Could you check a few things on this drawing? It's one solid part, dimensions in mm from its lowest x, y, z. A direction names the side the tool comes from. Give positions to 0.01 mm unless a question says otherwise; leave off trailing zeros. Order: outer loops, then holes, each group sorted by start corner. A loop starts at its lowest first (then second) coordinate and runs counter-clockwise, first axis right, second up.
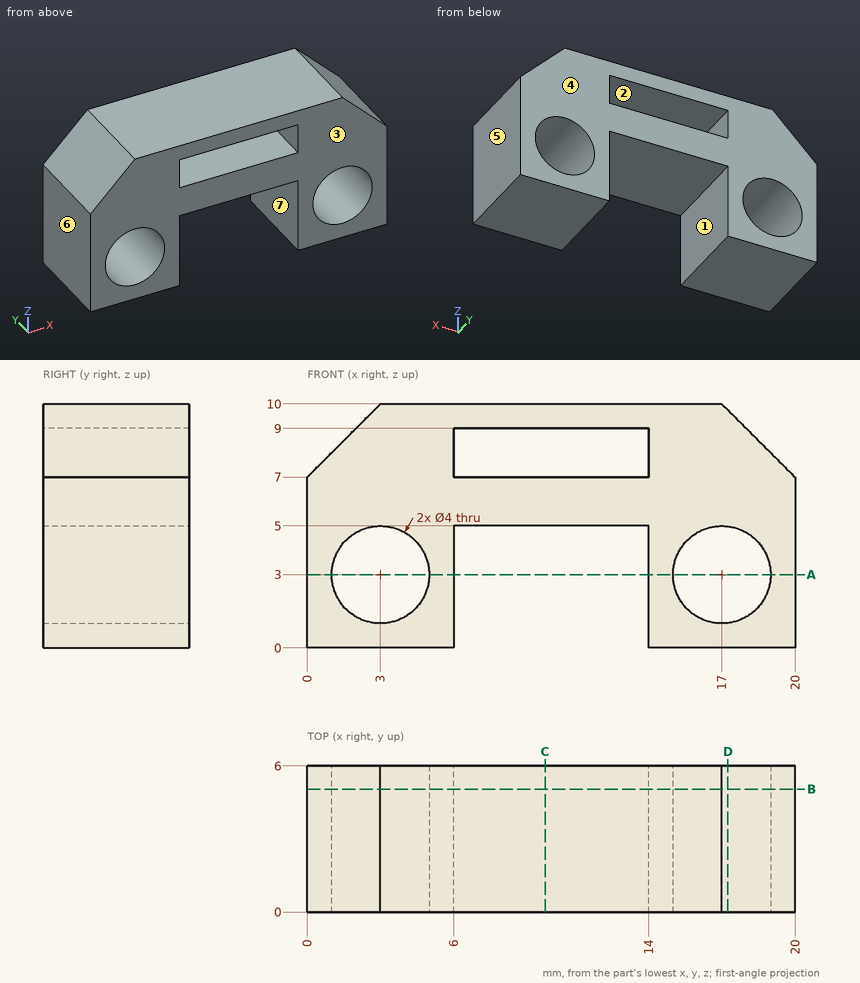
Q1. If we section it at C-C on x = 9.75: List the corners of the cut face in (y, z) for me.
Filled sheet:
outline: (0, 5) - (6, 5) - (6, 7) - (0, 7) - close; (0, 9) - (6, 9) - (6, 10) - (0, 10) - close
Q2. If we section it at D-D on x = 17.25: List the corners of the cut face in (y, z) for me.
Filled sheet:
outline: (0, 0) - (6, 0) - (6, 1.02) - (0, 1.02) - close; (0, 4.98) - (6, 4.98) - (6, 9.75) - (0, 9.75) - close
Q3. I'm going to push flat-ended pins straight in: P1, Ø0.6, axis at y = 4, z = 8, coming from the +X side; P2, Ø1.8, axis at x = 9, y = 2, coming from the -Z side; P3, Ø3, axis at x = 17, z = 3, coming from the +Y side. Where does each tip first touch, or does it pass through?
Filled sheet:
P1: stops at x = 19.3
P2: stops at z = 5
P3: passes through
Q4. If we section it at B-B on y = 5.05: List the corners of the cut face in (x, z) for me.
Filled sheet:
outline: (0, 0) - (6, 0) - (6, 5) - (14, 5) - (14, 0) - (20, 0) - (20, 7) - (17, 10) - (3, 10) - (0, 7) - close; hole circle Ø4 at (3, 3); hole (6, 7) - (14, 7) - (14, 9) - (6, 9) - close; hole circle Ø4 at (17, 3)
Q5. For the marked faces 1, 2 and 3, which set-ups out of +Z, -Z, +X, -X, +Y, -Y let a thin tool reach every point of the face, with its end or its side?
Filled sheet:
face 1: -Z, +Y, -Y
face 2: +Y, -Y
face 3: +Z, -Z, +X, -X, -Y
Q6. Thinking about a two-plate mould opening in X: for the marked faces 4, 5, 6 and 7, which applies, released by +X, released by -X, zero draft, split by the parting line, or undercut?
Filled sheet:
face 4: zero draft
face 5: released by +X
face 6: released by -X
face 7: undercut
Q7. If we section it at A-A on z = 3: List the corners of the cut face in (x, y) for me, plus the area to 3 significant figures.
Filled sheet:
outline: (0, 0) - (1, 0) - (1, 6) - (0, 6) - close; (5, 0) - (6, 0) - (6, 6) - (5, 6) - close; (14, 0) - (15, 0) - (15, 6) - (14, 6) - close; (19, 0) - (20, 0) - (20, 6) - (19, 6) - close
area: 24.0 mm2
Q8. I need wall thicknesses on L1, parallel to X at y = 4.6, z = 3; L2, parallel to X at y = 3.15, z = 4.75; L3, parallel to Z at x = 7.5, y = 3.85. Which ranges of each line are inside material? Lowest first, please.
Filled sheet:
L1: x = 0 to 1, 5 to 6, 14 to 15, 19 to 20
L2: x = 0 to 2.03, 3.97 to 6, 14 to 16.03, 17.97 to 20
L3: z = 5 to 7, 9 to 10
